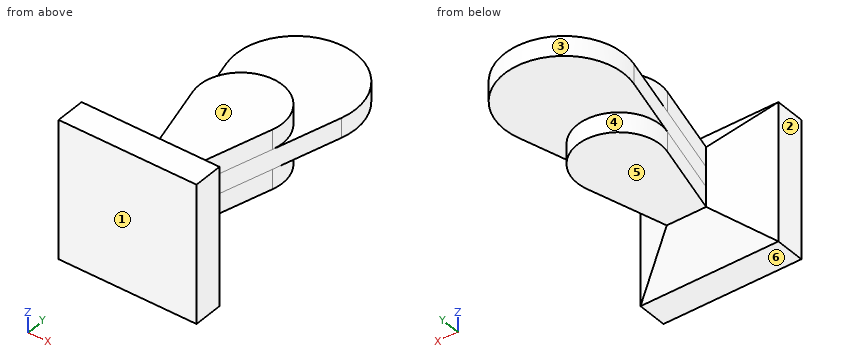
from build123d import *

# Parameters (mm, degrees)
SKETCH1_W      = 70
SKETCH1_H      = 70
EXTRUDE1_DEPTH = 15
SKETCH2_W      = 70
SKETCH2_H      = 70
SKETCH3_W      = 20
SKETCH3_H      = 30
EXTRUDE2_DEPTH = 5
EXTRUDE3_DEPTH = 15


with BuildPart() as part:
    # Sketch1 → Extrude1 (new body)
    with BuildSketch(Plane(origin=(0, 0, 0), x_dir=(1, 0, 0), z_dir=(0, 1, 0))):
        Rectangle(SKETCH1_W, SKETCH1_H)
    extrude(amount=EXTRUDE1_DEPTH)

    # Sketch2 → Loft1 section 0
    with BuildSketch(Plane(origin=(0, 15, 0), x_dir=(-1, 0, 0), z_dir=(0, 1, 0))):
        Rectangle(SKETCH2_W, SKETCH2_H)
    # Sketch3 → Loft1 section 1
    with BuildSketch(Plane(origin=(0, 30, 0), x_dir=(-1, 0, 0), z_dir=(0, 1, 0))):
        Rectangle(SKETCH3_W, SKETCH3_H)
    loft()

    # Sketch4 → Extrude2 (add, symmetric)
    with BuildSketch(Plane.XY):
        with BuildLine():
            Line((10, 30), (29.257681763, 101.870646776))
            ThreePointArc((29.257681763, 101.870646776), (0, 140), (-29.257681763, 101.870646776))
            Line((-29.257681763, 101.870646776), (-10, 30))
            Line((-10, 30), (10, 30))
        make_face()
    extrude(amount=EXTRUDE2_DEPTH, both=True)

    # Sketch5 → Extrude3 (add, symmetric)
    with BuildSketch(Plane.XY):
        with BuildLine():
            Line((20.320734039, 68.517503805), (10, 30))
            Line((10, 30), (-10, 30))
            Line((-10, 30), (-20.320734039, 68.517503805))
            ThreePointArc((-20.320734039, 68.517503805), (0, 95), (20.320734039, 68.517503805))
        make_face()
    extrude(amount=EXTRUDE3_DEPTH, both=True)


solid = part.part
Geometry: final body of the model. Coordinates: model frame, mm. Face numbers are marked on the shaded views. A direction names the side the tool comes from. Give positions to 0.01 mm unless a question says otherwise; leave off trailing zeros. Loops run counter-clockwise (first coordinate to the right, second up) from the corner with the lowest first, then second, coordinate; pieces in that order, holes last. Notation, with made-up numbers: (82, 60) - (104, 60) arc R8 ccw to (104, 70) - close; hole circle Ø7 at (20.25, 87.5). An arc over 180 degrees is marked (long way). Answer as CSV lines item,"result". Start each with the question number.
1. Section B-B, the plane y = 38. Return loops of the section in (x, z).
2. Reachability of the marked faces 4, 5, 6 and 7 from +Z, -Z, +X, -X, +Y, -Y: full face, straight path, thin tool, end or side. Return the list, or none.
3. Ray query, L1, parallel to Y at x = 1, z = -6; L2, parallel to Y at x = -1, z = -16; L3, parallel to Z at x = 9, y = 88. Return the intervals inside material, ascending.
4. Pin query (flat end, axial travel): P1, Ø18, axis at x = 3, y = 118, coming from the -Z side; P2, Ø1.5, axis at x = -15.5, y = 102, coming from the +Z side; P3, Ø21, axis at x = 2, y = 50.5, coming from the -Z side. Return the tip coordinate at first contact, or that it passes through.
5. Section A-A, the plane y = 81. Return loops of the section in (x, z).
6. Draft query along Y for the marked faces 1, 2 and 3. Return one class per face: released by +Y, released by -Y, zero draft, split by the parting line, or undercut.
Answers:
1,outline,"(-12.14, -15) - (12.14, -15) - (12.14, 15) - (-12.14, 15) - close"
2,face 4,"-Z"
2,face 5,"-Z, +X, -X, +Y"
2,face 6,"-Z, +X, -X, +Y, -Y"
2,face 7,"+Z, +X, -X, +Y"
3,L1,"y = 0 to 94.98"
3,L2,"y = 0 to 29.25"
3,L3,"z = -15 to 15"
4,P1,"stops at z = -5"
4,P2,"stops at z = 5"
4,P3,"stops at z = -15"
5,outline,"(-23.67, -5) - (-19.83, -5) - (-19.83, -15) - (19.83, -15) - (19.83, -5) - (23.67, -5) - (23.67, 5) - (19.83, 5) - (19.83, 15) - (-19.83, 15) - (-19.83, 5) - (-23.67, 5) - close"
6,face 1,"released by -Y"
6,face 2,"zero draft"
6,face 3,"undercut"
